Input: part model. Units: mm. Frame: model coordinates. A direction names the side the tool comes from. Coordinates: 2 decimals unless noted, no trailing zeros. Order: outer loops, then holes, each group sorted by start corner. A loop starts at its lowest first (then second) coordinate and runs counter-clockwise, first axis right, second up. Notation, with made-up numbers: M 75,5.25 L 103,5.25 A20 ccw 103,38.25 Z; hole C 59,-4.75 d4. An arc over 180 degrees is marked long. Answer in a Markdown table with one row per item.
from build123d import *

# Parameters (mm, degrees)
EXTRUDE1_DEPTH            = 32.5
SKETCH2_W                 = 70
SKETCH2_H                 = 1.7
CUT_EXTRUDE1_DEPTH        = 123.291955991
M5_CLEARANCE_HOLE1_D      = 5.5
M5X0_8_TAPPED_HOLE1_D     = 4.2
M5X0_8_TAPPED_HOLE1_DEPTH = 19.05
M5X0_8_TAPPED_HOLE1_TIP   = 1.2618073


with BuildPart() as part:
    # Sketch1 → Extrude1 (new, symmetric)
    with BuildSketch(Plane.XY):
        with BuildLine():
            Line((0, 0), (97, 0))
            Line((97, 0), (97, 12.7))
            Line((97, 12.7), (25.4, 12.7))
            ThreePointArc((25.4, 12.7), (16.419743879, 16.419743879), (12.7, 25.4))
            Line((12.7, 25.4), (12.7, 36.35))
            Line((12.7, 36.35), (0, 36.35))
            Line((0, 36.35), (0, 0))
        make_face()
    extrude(amount=EXTRUDE1_DEPTH, both=True)

    # Sketch2 → Cut-Extrude1 (cut, through all)
    with BuildSketch(Plane(origin=(0, 0, -32.5), x_dir=(-1, 0, 0), z_dir=(0, 0, -1))):
        with Locations((-62, 11.85)):
            Rectangle(SKETCH2_W, SKETCH2_H)
    extrude(amount=-CUT_EXTRUDE1_DEPTH, mode=Mode.SUBTRACT)

    # M5 Clearance Hole1 (through all)
    with Locations(Plane.XZ):
        with Locations((53.7, 15), (91.7, 15), (91.7, -15), (53.7, -15)):
            Hole(M5_CLEARANCE_HOLE1_D / 2)

    # M5x0.8 Tapped Hole1
    with Locations(Plane(origin=(0, 36.35, 0), x_dir=(-1, 0, 0), z_dir=(0, 1, 0))):
        with Locations((-6.35, 22.5), (-6.35, -22.5)):
            Hole(M5X0_8_TAPPED_HOLE1_D / 2, depth=M5X0_8_TAPPED_HOLE1_DEPTH)
            with Locations((0, 0, -(M5X0_8_TAPPED_HOLE1_DEPTH + M5X0_8_TAPPED_HOLE1_TIP / 2))):  # 118° drill point
                Cone(0, M5X0_8_TAPPED_HOLE1_D / 2, M5X0_8_TAPPED_HOLE1_TIP, mode=Mode.SUBTRACT)


solid = part.part
1) Mould query, pull axis X, two halves, no side actions, for faces 4 (the face through (89.08, 5.58, 15.83)), 5 (the face through (16.52, 16.32, 0.45)), 6 (the face through (62, 11, 0)). Classes: +X half, -X half, draft (parallel to the pull), parting line (faces both ways), or undercut.
Resolved:
| item | result |
|---|---|
| face 4 | undercut |
| face 5 | +X half |
| face 6 | draft |
2) Material intervals for probe 1 along Z at (x, y) = (91.7, 5.75); probe 2 along Z at (x, y) = (52, 1); probe 3 along Y at (x, z) = (35, 12.5), sorted ascending.
Resolved:
| item | result |
|---|---|
| probe 1 | z = -32.5 to -17.75, -12.25 to 12.25, 17.75 to 32.5 |
| probe 2 | z = -32.5 to -17.16, -12.84 to 12.84, 17.16 to 32.5 |
| probe 3 | y = 0 to 11 |
3) Cut plane A-A, the plane x = 53.7. Output: boundary loops of the cut face in (y, z).
Resolved:
| item | result |
|---|---|
| outline | M 0,-32.5 L 11,-32.5 L 11,-17.75 L 0,-17.75 Z; M 0,-12.25 L 11,-12.25 L 11,12.25 L 0,12.25 Z; M 0,17.75 L 11,17.75 L 11,32.5 L 0,32.5 Z |
4) Cut plane D-D, the plane y = 23. Output: boundary loops of the cut face in (x, z).
Resolved:
| item | result |
|---|---|
| outline | M 0,-32.5 L 12.93,-32.5 L 12.93,32.5 L 0,32.5 Z; hole C 6.35,-22.5 d4.2; hole C 6.35,22.5 d4.2 |
5) Cut plane B-B, the plane z = -15. Output: boundary loops of the cut face in (x, y), and give its area (3 significant figures).
Resolved:
| item | result |
|---|---|
| outline | M 0,0 L 50.95,0 L 50.95,11 L 27,11 L 27,12.7 L 25.4,12.7 A12.7 cw 12.7,25.4 L 12.7,36.35 L 0,36.35 Z; M 56.45,0 L 88.95,0 L 88.95,11 L 56.45,11 Z; M 94.45,0 L 97,0 L 97,11 L 94.45,11 Z |
| area | 1,330 mm2 |
6) Reachability of faces 1 (the face through (7.48, 26.69, -20.73)), 2 (the face through (37, 10, 32.5)), 3 (the face through (12.7, 31, 0)) from +Z, -Z, +X, -X, +Y, -Y: full face, straight path, thin tool, end or side. Return the list, or none.
Resolved:
| item | result |
|---|---|
| face 1 | +Y |
| face 2 | +Z, +X, -X, +Y, -Y |
| face 3 | +Z, -Z, +X, +Y |
7) Cut plane C-C, the plane z = -0.5. Output: boundary loops of the cut face in (x, y).
Resolved:
| item | result |
|---|---|
| outline | M 0,0 L 97,0 L 97,11 L 27,11 L 27,12.7 L 25.4,12.7 A12.7 cw 12.7,25.4 L 12.7,36.35 L 0,36.35 Z |
8) Contact query for flat-ended pins moving along their axis: pin 1 (4 mm diameter, centred on x = 6.35, z = -22.5, fed in from -Y); pin 2 (1 mm diameter, centred on y = 15.5, z = -3, fed in from +X); pin 3 (2 mm diameter, centred on y = 18, z = 23.5, fed in from +X); pin 4 (12 mm diameter, centred on y = 18.5, z = -16, fed in from +X). Output: stop coordinate, or through.
Resolved:
| item | result |
|---|---|
| pin 1 | stops at y = 0 |
| pin 2 | stops at x = 18.11 |
| pin 3 | stops at x = 15.87 |
| pin 4 | stops at x = 27 |
